Could you check a few things on this model? Use its own coordinates, in mm. Coordinates: 2 decimals unless noted, no trailing zeros. Write each loop counter-clockwise with the first axis right and the second up, starting at its lowest first coordinate (ties: lowest second). Pieces come first, ordered by that corner, then holes. Notation, with made-up numbers: M -28.5,36 L -12.5,36 A30 cw -12.5,60 Z; hole C 30,10 d4. An arc over 180 degrees is marked long. Answer as CSV lines item,"result". Start each with the question number.
Item 1: If I drill on line 1 along X through (y, z) = (1.45, -68); line 2 along X through (y, z) = (0.3, 59.5); line 3 along X through (y, z) = (1.4, 46.5), over which ranges is the centre line in solid material (lowest first)? Write a range as [from, to].
Item 2: We'd pull the mould along Z, two halves only. Please class faces 1 (the cylindrical face through (-106.422, 1.014, 46.162)), 2 (the cylindrical face through (111.58, 0.99, 45.94)), 3 (the flat face through (2, 2, -1)): +Z half, -Z half, draft (parallel to the pull), parting line (faces both ways), or undercut.
Item 3: Suppose I cut it at C-C, the plane z = 62. Write out the boundary of the cut face in (x, y).
Item 4: I'm going to push a flat-ended pin straight in: P1, Ø1, axis at x = -110, y = 1, coming from the +Z side. Where does the tip first touch, or does it pass through?
Item 5: Suppose I cut it at A-A, the plane x = 109. Write out the boundary of the cut face in (y, z).
Item 6: Suppose I cut it at B-B, the plane x = -109. Write out the boundary of the cut face in (y, z).
```python
from build123d import *

# Parameters (mm, degrees)
P_IDAT_VYSUNUT_M1_DEPTH  = 2
SKICA2_R                 = 2.6
ODEBRAT_VYSUNUT_M1_DEPTH = 2
SKICA3_R                 = 2.6
ODEBRAT_VYSUNUT_M2_DEPTH = 2


with BuildPart() as part:
    # Skica1 → Přidat vysunutím1 (new body)
    with BuildSketch(Plane(origin=(0, 0, 0), x_dir=(1, 0, 0), z_dir=(0, 1, 0))):
        Polygon((119, -76.5), (-99, -76.5), (-99, -56.5), (-119, -56.5), (-119, 76.5), (119, 76.5), align=None)
    extrude(amount=P_IDAT_VYSUNUT_M1_DEPTH)

    # Skica2 → Odebrat vysunutím1 (cut)
    with BuildSketch(Plane.XZ):
        with Locations(Location((109, 45.604467717, 0), (0, 0, 270))):
            Circle(SKICA2_R)
        with Locations(Location((109, -67.457548012, 0), (0, 0, 270))):
            Circle(SKICA2_R)
    extrude(amount=-ODEBRAT_VYSUNUT_M1_DEPTH, mode=Mode.SUBTRACT)

    # Skica3 → Odebrat vysunutím2 (cut)
    with BuildSketch(Plane(origin=(0, 2, 0), x_dir=(1, 0, 0), z_dir=(0, 1, 0))):
        with Locations(Location((-109, 66.5, 0), (0, 0, 270))):
            Circle(SKICA3_R)
        with Locations(Location((-109, -46.5, 0), (0, 0, 270))):
            Circle(SKICA3_R)
    extrude(amount=-ODEBRAT_VYSUNUT_M2_DEPTH, mode=Mode.SUBTRACT)


solid = part.part
```
Ans:
1,line 1,"x = [-119, -111.12], [-106.88, 106.46], [111.54, 119]"
1,line 2,"x = [-99, 119]"
1,line 3,"x = [-119, -111.6], [-106.4, 106.56], [111.44, 119]"
2,face 1,"undercut"
2,face 2,"undercut"
2,face 3,"draft"
3,outline,"M -99,0 L 119,0 L 119,2 L -99,2 Z"
4,P1,"stops at z = 56.5"
5,outline,"M 0,-76.5 L 2,-76.5 L 2,-70.06 L 0,-70.06 Z; M 0,-64.86 L 2,-64.86 L 2,43 L 0,43 Z; M 0,48.2 L 2,48.2 L 2,76.5 L 0,76.5 Z"
6,outline,"M 0,-76.5 L 2,-76.5 L 2,-69.1 L 0,-69.1 Z; M 0,-63.9 L 2,-63.9 L 2,43.9 L 0,43.9 Z; M 0,49.1 L 2,49.1 L 2,56.5 L 0,56.5 Z"
